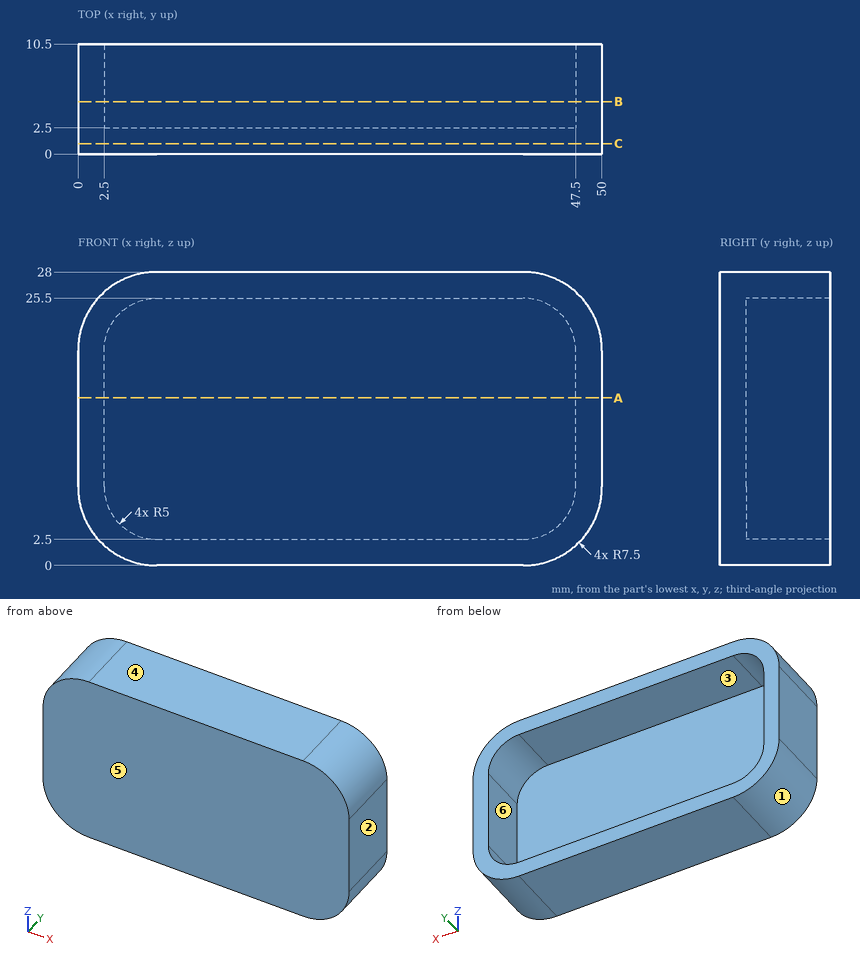
Source: three-view drawing plus pictorial views. Frame: mm from the lowest corner of the part. A direction names the side the tool comes from. Round coordinates to 2 decimals unless told otherwise and drop trailing zeros. Loops run counter-clockwise (first coordinate to the right, second up) from the corner with the lowest first, then second, coordinate; pieces in that order, holes last. Notation, with made-up numbers: M 57.25,15.25 L 78.25,15.25 A35 ccw 78.25,51.25 Z; hole C -4,89.5 d7. An arc over 180 degrees is marked long. Put each result on its own line as item: value. Start each with the question number.
(1) Draft query along Z for the marked faces 1, 2, 3 and 4. Return one class per face: +Z half, -Z half, draft (parallel to the pull), parting line (faces both ways), or undercut.
(2) Contact query for flat-ended pins moving along their axis: pin 1 Ø1.5 at (y, z) = (5, 6) entering from +X; pin 2 Ø8 at (x, z) = (37, 9) entering from +Y. Output: stop coordinate, or through.
(3) Section query B-B (y = 5). Return loops of the section in (x, z), then the cut area to 3 significant figures.
(4) Set-up query: the marked faces 5 and 6. Return all of +Z, -Z, +X, -X, +Y, -Y with unobstructed straight access to the full face (end or side cutting, diameter ignored); none if empty.
(5) Section query C-C (y = 1). Return loops of the section in (x, z), then the cut area to 3 significant figures.
(6) Material intervals for line 1 along Z through (x, y) = (34.5, 8.25); line 2 along X through (y, z) = (3.25, 14); line 3 along Y through (x, z) = (7, 21.25), sorted ascending. Write a range as [from, to].
(7) Section query A-A (z = 16). Return loops of the section in (x, y), then the cut area to 3 significant figures.
Findings below:
1. face 1: -Z half
1. face 2: draft
1. face 3: undercut
1. face 4: +Z half
2. pin 1: stops at x = 49.96
2. pin 2: stops at y = 2.5
3. outline: M 0,7.5 A7.5 ccw 7.5,0 L 42.5,0 A7.5 ccw 50,7.5 L 50,20.5 A7.5 ccw 42.5,28 L 7.5,28 A7.5 ccw 0,20.5 Z; hole M 2.5,7.5 A5 ccw 7.5,2.5 L 42.5,2.5 A5 ccw 47.5,7.5 L 47.5,20.5 A5 ccw 42.5,25.5 L 7.5,25.5 A5 ccw 2.5,20.5 Z
3. area: 338 mm2
4. face 5: +Z, -Z, +X, -X, -Y
4. face 6: +Y
5. outline: M 0,7.5 A7.5 ccw 7.5,0 L 42.5,0 A7.5 ccw 50,7.5 L 50,20.5 A7.5 ccw 42.5,28 L 7.5,28 A7.5 ccw 0,20.5 Z
5. area: 1,350 mm2
6. line 1: z = [0, 2.5], [25.5, 28]
6. line 2: x = [0, 2.5], [47.5, 50]
6. line 3: y = [0, 2.5]
7. outline: M 0,0 L 50,0 L 50,10.5 L 47.5,10.5 L 47.5,2.5 L 2.5,2.5 L 2.5,10.5 L 0,10.5 Z
7. area: 165 mm2
